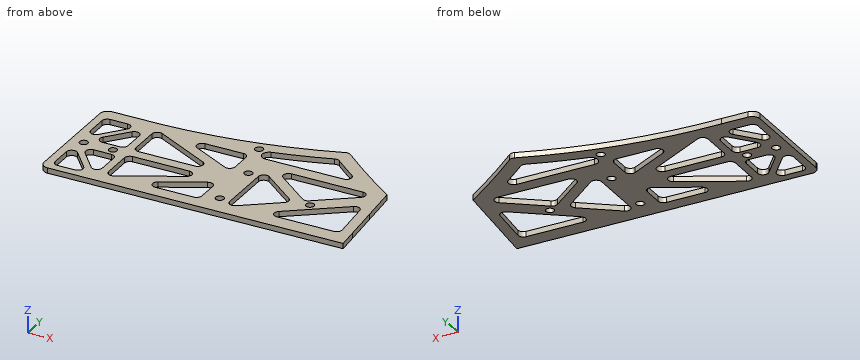
```python
from build123d import *

# Parameters (mm, degrees)
SKETCH_1_W           = 165
SKETCH_1_H           = 57
EXTRUDE_1_DEPTH      = 2
CUT_EXTRUDE_1_DEPTH  = 6
SKETCH_4_R           = 1.55
CUT_EXTRUDE_3_DEPTH  = 33
SKETCH_8_R           = 1.55
CUT_EXTRUDE_5_DEPTH  = 10
SKETCH_9_R           = 1.55
CUT_EXTRUDE_6_DEPTH  = 10
FILLET_3_R           = 2
FILLET_4_R           = 2
CUT_EXTRUDE_7_DEPTH  = 10
FILLET_8_R           = 2
CUT_EXTRUDE_8_DEPTH  = 10
FILLET_9_R           = 2
CUT_EXTRUDE_9_DEPTH  = 10
FILLET_10_R          = 2
EXTRUDE_4_DEPTH      = 2
FILLET_11_R          = 2
EXTRUDE_5_DEPTH      = 2
FILLET_12_R          = 2
CUT_EXTRUDE_10_DEPTH = 10
EXTRUDE_6_DEPTH      = 2
FILLET_13_R          = 3
SKETCH_18_R          = 1.55
CUT_EXTRUDE_12_DEPTH = 2
FILLET_14_R          = 2


with BuildPart() as part:
    # 草图1 → 凸台-拉伸1 (new body)
    with BuildSketch(Plane.XY):
        Rectangle(SKETCH_1_W, SKETCH_1_H)
    extrude(amount=EXTRUDE_1_DEPTH)

    # 草图2 → 切除-拉伸1 (cut)
    with BuildSketch(Plane.XY.offset(2)):
        with BuildLine():
            Line((82.5, 28.5), (-7.5, 28.5))
            ThreePointArc((-7.5, 28.5), (35.318614374, -3.444293093), (82.5, -28.5))
            Line((82.5, -28.5), (82.5, 28.5))
        make_face()
        with BuildLine():
            Line((-82.5, 28.5), (-82.5, 16.5))
            ThreePointArc((-82.5, 16.5), (-44.425115885, 18.906974283), (-7.5, 28.5))
            Line((-7.5, 28.5), (-82.5, 28.5))
        make_face()
    extrude(amount=-CUT_EXTRUDE_1_DEPTH, mode=Mode.SUBTRACT)

    # 草图4 → 切除-拉伸3 (cut)
    with BuildSketch(Plane.XY.offset(2)):
        with Locations((-77.5, -7)):
            Circle(SKETCH_4_R)
    extrude(amount=-CUT_EXTRUDE_3_DEPTH, mode=Mode.SUBTRACT)

    # 草图8 → 切除-拉伸5 (cut)
    with BuildSketch(Plane.XY.offset(2)):
        with Locations((-1.4, -10)):
            Circle(SKETCH_8_R)
        with Locations((-30.1, -20)):
            Circle(SKETCH_8_R)
        with Locations((-30.1, 0)):
            Circle(SKETCH_8_R)
    extrude(amount=-CUT_EXTRUDE_5_DEPTH, mode=Mode.SUBTRACT)

    # 草图9 → 切除-拉伸6 (cut)
    with BuildSketch(Plane(origin=(0, 0, 0), x_dir=(-1, 0, 0), z_dir=(0, 0, -1))):
        with Locations((35, 16.562431315)):
            Circle(SKETCH_9_R)
        with Locations((-40, -14.583150631)):
            Circle(SKETCH_9_R)
    extrude(amount=-CUT_EXTRUDE_6_DEPTH, mode=Mode.SUBTRACT)

    # 圆角3
    fillet_3_edges = [part.edges().sort_by_distance(p)[0] for p in [
        (-7.5, 28.5, 1),
    ]]
    fillet(fillet_3_edges, radius=FILLET_3_R)

    # 圆角4
    fillet_4_edges = [part.edges().sort_by_distance(p)[0] for p in [
        (-82.5, 16.5, 1),
        (-82.5, -28.5, 1),
    ]]
    fillet(fillet_4_edges, radius=FILLET_4_R)

    # 草图10 → 切除-拉伸7 (cut)
    with BuildSketch(Plane.XY.offset(2)):
        with BuildLine():
            Line((-29.849630584, 11.395100666), (5.446787044, 11.395100666))
            ThreePointArc((5.446787044, 11.395100666), (-1.632648985, 17.014079013), (-8.566742511, 22.811464555))
            ThreePointArc((-8.566742511, 22.811464555), (-19.410140236, 19.367286283), (-30.427912484, 16.529975425))
            ThreePointArc((-30.427912484, 16.529975425), (-32.433297975, 13.704131917), (-29.849630584, 11.395100666))
        make_face()
    extrude(amount=-CUT_EXTRUDE_7_DEPTH, mode=Mode.SUBTRACT)

    # 圆角8
    fillet_8_edges = [part.edges().sort_by_distance(p)[0] for p in [
        (-8.566742511, 22.811464555, 1),
        (5.446787044, 11.395100666, 1),
    ]]
    fillet(fillet_8_edges, radius=FILLET_8_R)

    # 草图11 → 切除-拉伸8 (cut)
    with BuildSketch(Plane.XY.offset(2)):
        Polygon((-36.1, -23.450877229), (-60.842981063, -23.450877229), (-36.1, -10.539715916), align=None)
        Polygon((-39.932804883, -8.027888281), (-71.5, -8.027888281), (-71.5, -24.5), align=None)
        Polygon((-39.932804883, -4.027888281), (-71.5, 12.444223438), (-71.5, -4.027888281), align=None)
        Polygon((-36.1, -1.516060646), (-36.1, 11.395100666), (-60.842981063, 11.395100666), align=None)
    extrude(amount=-CUT_EXTRUDE_8_DEPTH, mode=Mode.SUBTRACT)

    # 圆角9
    fillet_9_edges = [part.edges().sort_by_distance(p)[0] for p in [
        (-39.932804883, -8.027888281, 1),
        (-71.5, -24.5, 1),
        (-71.5, -8.027888281, 1),
        (-39.932804883, -4.027888281, 1),
        (-71.5, -4.027888281, 1),
        (-71.5, 12.444223438, 1),
        (-36.1, 11.395100666, 1),
        (-36.1, -1.516060646, 1),
        (-60.842981063, 11.395100666, 1),
        (-36.1, -23.450877229, 1),
        (-60.842981063, -23.450877229, 1),
        (-36.1, -10.539715916, 1),
    ]]
    fillet(fillet_9_edges, radius=FILLET_9_R)

    # 草图12 → 切除-拉伸9 (cut)
    with BuildSketch(Plane.XY.offset(2)):
        with BuildLine():
            Line((-26.1, 6.395100666), (-26.1, -24.5))
            Line((-26.1, -24.5), (10.872926165, 2.785876305))
            ThreePointArc((10.872926165, 2.785876305), (11.585120693, 5.020221166), (9.68532482, 6.395100666))
            Line((9.68532482, 6.395100666), (-26.1, 6.395100666))
        make_face()
        with BuildLine():
            Line((16.519718688, -0.503821347), (-13.285557865, -22.5))
            Line((-13.285557865, -22.5), (51.996010319, -22.5))
            ThreePointArc((51.996010319, -22.5), (33.937003057, -12.019408482), (16.519718688, -0.503821347))
        make_face()
    extrude(amount=-CUT_EXTRUDE_9_DEPTH, mode=Mode.SUBTRACT)

    # 圆角10
    fillet_10_edges = [part.edges().sort_by_distance(p)[0] for p in [
        (16.519718688, -0.503821347, 1),
        (51.996010319, -22.5, 1),
        (-13.285557865, -22.5, 1),
        (-26.1, 6.395100666, 1),
        (-26.1, -24.5, 1),
    ]]
    fillet(fillet_10_edges, radius=FILLET_10_R)

    # 草图13 → 凸台-拉伸4 (add)
    with BuildSketch(Plane.XY.offset(2)):
        Polygon((-26.758433391, 4.243454395), (-7.263956073, -11.246702958), (-4.352943402, -8.450756462), (-24.269993734, 7.375174063), align=None)
    extrude(amount=-EXTRUDE_4_DEPTH)

    # 圆角11
    fillet_11_edges = [part.edges().sort_by_distance(p)[0] for p in [
        (-26.1, 3.720268435, 1),
        (-7.686529087, -10.910929786, 1),
        (-4.352943402, -8.450756462, 1),
        (-23.036564134, 6.395100666, 1),
    ]]
    fillet(fillet_11_edges, radius=FILLET_11_R)

    # 草图14 → 凸台-拉伸5 (add)
    with BuildSketch(Plane.XY.offset(2)):
        Polygon((14.53207819, -1.153752135), (16.546586595, -22.68629933), (20.546624568, -22.5), (18.514686662, -0.781153475), align=None)
    extrude(amount=-EXTRUDE_5_DEPTH)

    # 圆角12
    fillet_12_edges = [part.edges().sort_by_distance(p)[0] for p in [
        (14.603571968, -1.917930204, 1),
        (16.529157093, -22.5, 1),
        (20.546624568, -22.5, 1),
        (18.626422966, -1.975473255, 1),
    ]]
    fillet(fillet_12_edges, radius=FILLET_12_R)

    # 草图15 → 切除-拉伸10 (cut)
    with BuildSketch(Plane.XY.offset(2)):
        with BuildLine():
            Line((21.107963193, -28.5), (17.644547538, 8.519533342))
            ThreePointArc((17.644547538, 8.519533342), (49.082122431, -11.724904385), (82.5, -28.5))
            Line((82.5, -28.5), (21.107963193, -28.5))
        make_face()
    extrude(amount=-CUT_EXTRUDE_10_DEPTH, mode=Mode.SUBTRACT)

    # 草图17 → 凸台-拉伸6 (add)
    with BuildSketch(Plane.XY.offset(2)):
        Polygon((-80.455675407, 16.444223438), (-93.5, 16.444223438), (-93.5, -28.5), (-80.442860064, -28.5), align=None)
    extrude(amount=-EXTRUDE_6_DEPTH)

    # 圆角13
    fillet_13_edges = [part.edges().sort_by_distance(p)[0] for p in [
        (-93.5, -28.5, 1),
        (-93.5, 16.444223438, 1),
    ]]
    fillet(fillet_13_edges, radius=FILLET_13_R)

    # 草图18 → 切除-拉伸12 (cut)
    with BuildSketch(Plane.XY.offset(2)):
        with Locations((-88.5, -7)):
            Circle(SKETCH_18_R)
        Polygon((-74.5, -4), (-87.418023291, -4), (-74.5, 11.395100666), align=None)
        Polygon((-90.5, 11.395100666), (-90.5, -4), (-77.581976709, 11.395100666), align=None)
        Polygon((-87.418023291, -10), (-74.5, -25.395100666), (-74.5, -10), align=None)
        Polygon((-90.5, -10), (-77.581976709, -25.395100666), (-90.5, -25.395100666), align=None)
    extrude(amount=-CUT_EXTRUDE_12_DEPTH, mode=Mode.SUBTRACT)

    # 圆角14
    fillet_14_edges = [part.edges().sort_by_distance(p)[0] for p in [
        (-87.418023291, -10, 1),
        (-74.5, -10, 1),
        (-74.5, -25.395100666, 1),
        (-90.5, -25.395100666, 1),
        (-90.5, -10, 1),
        (-77.581976709, -25.395100666, 1),
        (-74.5, 11.395100666, 1),
        (-74.5, -4, 1),
        (-87.418023291, -4, 1),
        (-90.5, 11.395100666, 1),
        (-77.581976709, 11.395100666, 1),
        (-90.5, -4, 1),
    ]]
    fillet(fillet_14_edges, radius=FILLET_14_R)


solid = part.part
```
Could you check a few things on this model? Use its own coordinates, in mm. Round coordinates to 2 decimals unless told otherwise and drop trailing zeros. Loops run counter-clockwise (first coordinate to the right, second up) from the corner with the lowest first, then second, coordinate; pieces in that order, holes last.
Q1. I want a section at A-A (x = -35). Write out the boundary of the cut face in (y, z), and give its area (3 significant figures).
Q2. For P1, Ø1, axis at y = -10.5, z = 0.5, coming from the +X side; P2, Ø1, axis at y = 10.5, z = 1.5, coming from the +X side; P3, Ø0.6, axis at y = -21, z = 1, coming from the +X side, each with a flat end and sliding along its axis, tell me the tip position at first contact or that it passes through.
Q3. Please list where these lines run through material, in increasing order: L1, parallel to Y at x = -88.5, z = 0.7; L2, parallel to X at y = 7, z = 1.9; L3, parallel to Y at x = -75, z = 0.95.
Q4. I want a section at B-B (x = 4.5). Write out the boundary of the cut face in (y, z).
Q5. I want a section at C-C (x = -51.5). Write out the boundary of the cut face in (y, z).
Answer below:
1. outline: (-28.5, 0) - (15.01, 0) - (15.01, 2) - (-28.5, 2) - close; (18.11, 0) - (20.65, 0) - (20.65, 2) - (18.11, 2) - close
1. area: 92.1 mm2
2. P1: stops at x = 19.47
2. P2: stops at x = 15.61
2. P3: stops at x = 20.43
3. L1: y = -28.5 to -25.4, -13.49 to -8.55, -5.45 to -0.51, 11.4 to 16.44
3. L2: x = -93.5 to -90.5, -81.27 to -78.19, -74.83 to -71.5, -61.07 to -52.42, -36.1 to 17.79
3. L3: y = -28.5 to -21.22, -10.68 to -3.32, 7.22 to 16.4
4. outline: (-28.5, 0) - (-22.5, 0) - (-22.5, 2) - (-28.5, 2) - close; (-9.37, 0) - (-1.92, 0) - (-1.92, 2) - (-9.37, 2) - close; (6.4, 0) - (18.49, 0) - (18.49, 2) - (6.4, 2) - close
5. outline: (-28.5, 0) - (-23.45, 0) - (-23.45, 2) - (-28.5, 2) - close; (-18.58, 0) - (-14.06, 0) - (-14.06, 2) - (-18.58, 2) - close; (-8.03, 0) - (-4.03, 0) - (-4.03, 2) - (-8.03, 2) - close; (2.01, 0) - (6.52, 0) - (6.52, 2) - (2.01, 2) - close; (11.4, 0) - (17.9, 0) - (17.9, 2) - (11.4, 2) - close
